from build123d import *

# Parameters (mm, degrees)
SKETCH2_R           = 7.5
BOSS_EXTRUDE1_DEPTH = 5
BOSS_EXTRUDE1_TAPER = 10
SKETCH3_R           = 7.5
BOSS_EXTRUDE2_DEPTH = 1
FILLET1_R           = 1


with BuildPart() as part:
    # Sketch2 → Boss-Extrude1 (new body)
    with BuildSketch(Plane(origin=(0, 0, 0), x_dir=(1, 0, 0), z_dir=(0, 1, 0))):
        Circle(SKETCH2_R)
    extrude(amount=-BOSS_EXTRUDE1_DEPTH, taper=BOSS_EXTRUDE1_TAPER)

    # Sketch3 → Boss-Extrude2 (add)
    with BuildSketch(Plane(origin=(0, 0, 0), x_dir=(1, 0, 0), z_dir=(0, 1, 0))):
        Circle(SKETCH3_R)
    extrude(amount=BOSS_EXTRUDE2_DEPTH)

    # Fillet1
    fillet1_edges = [part.edges().sort_by_distance(p)[0] for p in [
        (-7.5, 0, 0),
        (-6.618365096, -5, 0),
    ]]
    fillet(fillet1_edges, radius=FILLET1_R)


solid = part.part
Here's how the part is built. I have some questions about the finished solid (model axes, mm). Give positions to 0.01 mm unless a question says otherwise; leave off trailing zeros. Order: outer loops, then holes, each group sorted by start corner. A loop starts at its lowest first (then second) coordinate and runs counter-clockwise, first axis right, second up. Notation, with made-up numbers: M 34.25,-7.5 L 69.25,-7.5 A21 cw 69.25,27.5 Z; hole C -37.75,-37.75 d6. An arc over 180 degrees is marked long. Answer as a JSON object with one key per item and string values. Group by question number.
1) Suppose I cut it at B-B, the plane y = -1.5. Write out the boundary of the cut face in (x, z), plus the area to 3 significant figures.
2) I'm going to push flat-ended pins straight in: pin 1 Ø2 at (x, z) = (5, 5) entering from -Y; pin 2 Ø1.5 at (y, z) = (-2.5, 6) entering from -X; pin 3 Ø1 at (x, y) = (1.5, 0.5) entering from +Z. Where does each tip first touch, or does it pass through?
3) Please list where these lines run through material, in increasing order: L1, parallel to Z at x = -0.25, y = 0.5; L2, parallel to Z at x = 1.25, y = -2; L3, parallel to X at y = -2, z = -5.25. Write a range as [from, to].
4) Suppose I cut it at A-A, the plane y = -2.75. Write out the boundary of the cut face in (x, z).
Results found:
{
 "1": {"outline": "C 0,0 d14.47", "area": "164 mm²"},
 "2": {"pin 1": "y = -4.96", "pin 2": "x = -4.74", "pin 3": "z = 7.43"},
 "3": {"L1": "[-7.5, 7.5]", "L2": "[-7.04, 7.04]", "L3": "[-4.85, 4.85]"},
 "4": {"outline": "C 0,0 d14.03"}
}
